Verification items for the finished model (mm, model axes). A direction names the side the tool comes from. Round coordinates to 2 decimals unless told otherwise and drop trailing zeros. Write each loop counter-clockwise with the first axis right and the second up, starting at its lowest first coordinate (ties: lowest second). Pieces come first, ordered by that corner, then holes. Notation, with made-up numbers: M 27.25,-6 L 45.25,-6 A12 cw 45.25,0 Z; hole C -17,80 d7. An arc over 180 degrees is marked long. Write each question's results on one line, items separated by ' | '.
from build123d import *

# Parameters (mm, degrees)
F5_DEPTH = 4
F7_D     = 3
F8_D     = 3


with BuildPart() as f5:
    # F4 (on Top) → F5 (new body)
    with BuildSketch(Plane.XY):
        Polygon((31.7157287525, 60), (-31.7157287525, 60), (-45.8578643763, 45.8578643763), (-60, 31.7157287525), (-53.459262274, 24.1143308548), (-52.5, 22.9995125363), (-52.5, -22.9995125363), (-60, -31.7157287525), (-45.8578643763, -45.8578643763), (-31.7157287525, -60), (31.7157287525, -60), (45.8578643763, -45.8578643763), (60, -31.7157287525), (52.5, -22.9995125363), (52.5, 22.9995125363), (60, 31.7157287525), (45.8578643763, 45.8578643763), align=None)
    extrude(amount=F5_DEPTH)

    # F7 (through all)
    with Locations(Plane.XY.offset(4)):
        with Locations((-40.75, 0), (40.75, -8), (40.75, 8)):
            Hole(F7_D / 2)

    # F8 (through all)
    with Locations(Plane(origin=(0, 0, 0), x_dir=(1, 0, 0), z_dir=(0, 0, -1))):
        with Locations((-49.3933982822, -35.2512626585), (-35.2512626585, -49.3933982822), (35.5175525155, -49.6500174851), (49.1271084251, -34.9946434556), (49.3933982822, 35.2512626585), (35.2512626585, 49.3933982822), (-35.2512626585, 49.3933982822), (-49.3933982822, 35.2512626585)):
            Hole(F8_D / 2)


solid = f5.part
1) Sectioned sample at B-B, the plane x = 40.75. Record the cut outline in (y, z).
Calculated:
outline: M -50.97,0 L -9.5,0 L -9.5,4 L -50.97,4 Z; M -6.5,0 L 6.5,0 L 6.5,4 L -6.5,4 Z; M 9.5,0 L 50.97,0 L 50.97,4 L 9.5,4 Z
2) Access from +Z, -Z, +X, -X, +Y, -Y to the whole of each face (thin tool, end or side, straight path). Record for faces 1 (the flat face through (56.302, -27.419, 1.972)), 2 (the cylindrical face through (34.56, -48.06, 2.03)), 3 (the flat face through (-52.5, 0, 2)).
Calculated:
face 1: +Z, -Z, +X | face 2: +Z, -Z | face 3: +Z, -Z, -X
3) Sectioned sample at D-D, the plane z = 1.6. Count the separate pieces of the cut face and the enclosed holes in it, and give its area (3 significant figures).
Calculated:
separate pieces: 1 | enclosed holes: 11 | area: 11,900 mm²
4) Sectioned sample at C-C, the plane x = -40.75. Record the cut outline in (y, z), and give its area (3 significant figures).
Calculated:
outline: M -50.97,0 L -1.5,0 L -1.5,4 L -50.97,4 Z; M 1.5,0 L 50.97,0 L 50.97,4 L 1.5,4 Z | area: 396 mm²
5) Draft check along Y on faces 4 (the flat face through (0, 60, 2)), 5 (the flat face through (-1, 1, 4)), 6 (the cylindrical face through (36.71, 50.56, 2.03)). Enter one of: pulls with the +Y half, pulls with the -Y half, needs draft (parallel to the pull), parting line crosses it, or undercut.
Calculated:
face 4: pulls with the +Y half | face 5: needs draft | face 6: undercut
6) Depth check by flat-ended pin: P1, Ø2.5, axis at x = 49.13, y = 34.99, coming from the +Z side; P2, Ø1.5, axis at x = 39.5, z = 3, coming from the -Y side. Enter the tip coordinate at first touch or a pass-through.
Calculated:
P1: passes through | P2: stops at y = -52.97
7) Sectioned sample at A-A, the plane y = 8. Record the cut outline in (x, z), and give its area (3 significant figures).
Calculated:
outline: M -52.5,0 L 39.25,0 L 39.25,4 L -52.5,4 Z; M 42.25,0 L 52.5,0 L 52.5,4 L 42.25,4 Z | area: 408 mm²
8) Material ranges on line 1 (X direction, y = 49.5, z = 1.9); line 2 (X direction, y = -23, z = 1.7); line 3 (Y direction, x = 40.75, z = 1.2), recorded low to high. Write a range as [from, to].
Calculated:
line 1: x = [-42.22, -36.75], [-33.76, 34.03], [37.01, 42.22] | line 2: x = [-52.5, 52.5] | line 3: y = [-50.97, -9.5], [-6.5, 6.5], [9.5, 50.97]
